Autodesk Inventor part; units mm, degrees
ref_plane "YZ Plane" through (0, 0, 0) normal (1, 0, 0) x (0, 1, 0)
ref_plane "XZ Plane" through (0, 0, 0) normal (0, 1, 0) x (-1, 0, 0)
ref_plane "XY Plane" through (0, 0, 0) normal (0, 0, 1) x (1, 0, 0)
sketch "Sketch1" plane through (0, 0, 0) normal (0, 0, 1) x (1, 0, 0)
  line L0 (17, 4.5) -> (17, -4.5)
  line L1 (-17, -4.5) -> (-17, 4.5)
  arc A0 (-8.3666, -4.5) -> (8.3666, -4.5) centre (0, 0) ccw
  arc A1 (8.3666, 4.5) -> (-8.3666, 4.5) centre (0, 0) ccw
  line L2 (-17, 4.5) -> (-8.3666, 4.5)
  line L3 (8.3666, 4.5) -> (17, 4.5)
  line L4 (17, -4.5) -> (8.3666, -4.5)
  line L5 (-8.3666, -4.5) -> (-17, -4.5)
  line L6 (-17, 4.5) -> (17, -4.5) construction
  line L7 (-17, -4.5) -> (17, 4.5) construction
  point P0 (0, 0)
  point P1 (0, 0)
  dimension "d0" = 9
  dimension "d1" = 34
  dimension "d2" = 9.5
  dimension "d3" = 9
  dimension "d4" = 9.5
  dimension "d12" = 4.5
extrude "Extrusion1" add sketch "Sketch1" along normal blind 7
sketch "Sketch2" plane through (17, -4.5, 0) normal (1, 0, 0) x (0, 0, -1)
  arc A0 (-11.5, 9) -> (-11.5, 0) centre (-11.5, 4.5) ccw
  circle A1 centre (-11.5, 4.5) radius 2.25
  line L0 (-7, 9) -> (-11.5, 9)
  line L1 (-11.5, 0) -> (-7, 0)
  line L2 (-7, 0) -> (-7, 9)
  point P0 (0, 4.5)
  point P1 (-7, 0)
  dimension "d7" = 9
  dimension "d8" = 4.5
  dimension "d9" = 9
extrude "Extrusion2" add sketch "Sketch2" against normal blind 4.3
extrude "Extrusion3" add sketch "Sketch2" along normal blind 4.3 from surface at -34
sketch "Sketch3" plane through (-17, -4.5, 0) normal (0, -1, 0) x (1, 0, 0)
  line L0 (0, 6) -> (0, 0)
  line L1 (0, 0) -> (5, 0)
  line L2 (5, 0) -> (0, 6)
  line L3 (29, 0) -> (34, 0)
  line L4 (34, 0) -> (34, 6)
  line L5 (34, 6) -> (29, 0)
  point P0 (17, 0)
  dimension "d15" = 6
  dimension "d16" = 5
  dimension "d17" = 6
  dimension "d18" = 5
extrude "Extrusion4" cut sketch "Sketch3" against normal up to next
sketch "Sketch4" plane through (0, 0, 0) normal (0, 0, -1) x (-1, 0, 0)
  circle A0 centre (0, 0) radius 7.5
  dimension "d21" = 15
extrude "Extrusion5" add sketch "Sketch4" along normal blind 2.5
sketch "Sketch5" plane through (0, 0, 7) normal (0, 0, 1) x (1, 0, 0)
  circle A0 centre (0, 0) radius 7.5
  dimension "d24" = 15
extrude "Extrusion6" cut sketch "Sketch5" against normal blind 4
sketch "Sketch6" plane through (0, 0, -2.5) normal (0, 0, -1) x (-1, 0, 0)
  circle A0 centre (0, 0) radius 5.5
  dimension "d27" = 11
extrude "Extrusion7" cut sketch "Sketch6" against normal blind 4
sketch "Sketch7" plane through (0, 0, 1.5) normal (0, 0, -1) x (-1, 0, 0)
  circle A0 centre (0, 0) radius 5
  dimension "d30" = 10
extrude "Extrusion8" cut sketch "Sketch7" against normal up to next
sketch "Sketch9" plane through (0, 0, 0) normal (1, 0, 0) x (0, 1, 0)
  arc A0 (31.2893, 14.3034) -> (30.2107, 19.6966) centre (30.75, 17) ccw
  line L0 (-9.5504, 0) -> (57.3026, 0)
  line L1 (0, -37.6235) -> (0, 29.8791)
  circle A1 centre (30.75, 17) radius 1.25
  arc A2 (25.2107, 18.6966) -> (23.9154, 18.0486) centre (25.75, 16) ccw
  circle A3 centre (25.75, 16) radius 1.25
  line L2 (9.5, 7) -> (9.5, 0)
  line L3 (9.5, 0) -> (12.3425, 0)
  line L4 (25.2107, 18.6966) -> (30.2107, 19.6966)
  line L5 (26.2893, 13.3034) -> (31.2893, 14.3034)
  arc A4 (23.9154, 18.0486) -> (9.5, 7) centre (47.7522, -27.9802) ccw
  arc A5 (26.2893, 13.3034) -> (14.061, 0.9769) centre (44.8843, -17.3723) ccw
  arc A6 (12.3425, 0) -> (14.061, 0.9769) centre (12.3425, 2) ccw
  line L6 (8.5, 7) -> (9.5, 7)
  line L7 (9.5, 7) -> (9.5, 0)
  line L8 (9.5, 0) -> (8.5, 0)
  line L9 (8.5, 0) -> (8.5, 7)
  point P0 (0, 0)
  point P1 (13.5, 0)
  dimension "d53" = 5.5
  dimension "d54" = 17
  dimension "d55" = 30.75
  dimension "d56" = 2.5
  dimension "d57" = 16
  dimension "d58" = 25.75
  dimension "d59" = 4
  dimension "d60" = 7
  dimension "d61" = 9.5
  dimension "d62" = 0
  dimension "d63" = 51.8348
  dimension "d64" = 35.8716
  dimension "d65" = 2
  dimension "d88" = 7
  dimension "d89" = 1
  dimension "d90" = 0
  dimension "d91" = 0
extrude "Extrusion9" add sketch "Sketch9" along normal mid plane 4 contours L5 A5 A6 L0 L2 A4 A2 L4 A0
sketch "Sketch10" plane through (0, 0, 0) normal (1, 0, 0) x (0, 1, 0)
  arc A0 (25.2107, 18.6966) -> (26.2893, 13.3034) centre (25.75, 16) ccw
  circle A1 centre (25.75, 16) radius 1.25
  arc A2 (31.2893, 14.3034) -> (30.2107, 19.6966) centre (30.75, 17) ccw
  circle A3 centre (25.75, 16) radius 1.25
  circle A4 centre (30.75, 17) radius 1.25
  circle A5 centre (30.75, 17) radius 1.25
  line L0 (25.2107, 18.6966) -> (30.2107, 19.6966)
  line L1 (26.2893, 13.3034) -> (31.2893, 14.3034)
  point P0 (0, 0)
  dimension "d68" = 5.5
  dimension "d69" = 2.5
extrude "Extrusion10" add sketch "Sketch10" against normal blind 3.5
sketch "Sketch11" plane through (0, 0, 0) normal (1, 0, 0) x (0, 1, 0)
  line L0 (-4.2102, 0) -> (25.2612, 0)
  line L1 (0, -2.5102) -> (0, 15.0612)
  line L2 (19.9196, 12.551) -> (11.6686, 4.3)
  line L3 (11.6686, 4.3) -> (0, 4.3)
  line L4 (21.051, 11.4196) -> (12.3314, 2.7)
  line L5 (12.3314, 2.7) -> (0, 2.7)
  line L6 (21.051, 11.4196) -> (19.9196, 12.551)
  line L7 (0, 4.3) -> (0, 2.7)
  point P0 (0, 0)
extrude "Extrusion11" add sketch "Sketch11" along normal mid plane 12
extrude "Extrusion12" cut sketch "Sketch5" against normal blind 4
extrude "Extrusion13" cut sketch "Sketch7" against normal through all
sketch "Sketch12" plane through (0, 0, 0) normal (0, 0, 1) x (1, 0, 0)
  line L0 (6, 7.3655) -> (6, 12.3314)
  line L1 (2, 21.051) -> (6, 21.051)
  arc A0 (6, 7.3655) -> (2, 21.051) centre (-49.0316, -1.2919) ccw
  line L2 (0, 0) -> (0, 16.5543) construction
  arc A1 (-2, 21.051) -> (-6, 7.3655) centre (49.0316, -1.2919) ccw
  line L3 (2, 26.2893) -> (2, 14.061) construction
  line L4 (2, 21.051) -> (6, 21.051)
  line L5 (6, 7.3655) -> (6, 21.051)
  line L6 (-6, 7.3655) -> (-6, 21.051)
  line L7 (-2, 21.051) -> (-6, 21.051)
extrude "Extrusion14" cut sketch "Sketch12" along normal up to next
sketch "Sketch13" plane through (0, 0, 0) normal (1, 0, 0) x (0, 1, 0)
  line L0 (8.5, 7) -> (9.5, 7)
  line L1 (9.5, 7) -> (9.5, 0)
  line L2 (9.5, 0) -> (8.5, 0)
  line L3 (8.5, 0) -> (8.5, 7)
  line L4 (0, -6.95) -> (0, 24.2)
  line L5 (-18.1, 0) -> (42.1, 0)
  point P0 (0, 0)
  dimension "d92" = 7
  dimension "d93" = 1
  dimension "d94" = 9.5
  dimension "d95" = 0
extrude "Extrusion15" add sketch "Sketch13" along normal mid plane 4
properties part number "RCT-P006_steering_knuckle"
Geometry check sheet. Reference: the model listing, model coordinates, mm. A direction names the side the tool comes from. Coordinates: 2 decimals unless noted, no trailing zeros. Loops run counter-clockwise (first coordinate to the right, second up) from the corner with the lowest first, then second, coordinate; pieces in that order, holes last. Notation, with made-up numbers: (57.25, 17) - (107.25, 17) arc R24 ccw to (107.25, 49) - close; hole circle Ø9 at (-16.75, -16). An arc over 180 degrees is marked (long way). One line per item, written item: value. Start each with the question number.
(1) Tool access check on faces 1 (the cylindrical face through (-6.454, 6.971, 3.451)), 2 (the flat face through (-13, 4.5, 6)), 3 (the flat face through (6, 5, 0)), 4 (the flat face through (13, 4.5, 6)), 5 (the flat face through (-3.25, 14.94, 7.57)). Record the directions out of +Z, -Z, +X, -X, +Y, -Y that give a thin tool (end or side, any length) a straight path to the whole face; none if there is none.
(2) Cross-section at C-C on x = -14. Enter the section's corners in (y, z), plus the area to 3 significant figures.
(3) Material ranges on line 1 (Y direction, x = 0, z = -1); line 2 (Y direction, x = -13.6, z = 11.5); line 3 (X direction, y = 1.5, z = 8.5), recorded low to high. Write a range as [from, to].
(4) Cross-section at D-D on y = 25.75. Enter the section's corners in (x, z).
(5) Cross-section at B-B on x = 0. Enter the section's corners in (y, z).
(6) Mould release check, pull along Y, two halves, no side actions. Record for faces 6 (the cylindrical face through (-0.788, 26.422, 14.946)), 7 (the cylindrical face through (4.279, 14.876, 6.873)), 8 (the flat face through (-0.71, 27.68, 19.19)): released by +Y, released by -Y, zero draft, split by the parting line, or undercut.
(7) Cross-section at A-A on y = 0. Count the separate pieces of the cut face and the enclosed holes in it, plus the area to 3 significant figures.
(8) Depth check by flat-ended pin: P1, Ø10, axis at x = 2.5, z = 16.5, coming from the -Y side; P2, Ø12, axis at y = 25, z = 16, coming from the +X side; P3, Ø7, axis at x = -12.5, z = 3.5, coming from the +Y side. Enter the tip coordinate at first touch or a pass-through.
Results below:
1. face 1: -X
1. face 2: +Z, -Z, -X, +Y
1. face 3: -Z
1. face 4: +Z, -Z, +X, +Y
1. face 5: +Z, -X
2. outline: (-4.5, 2.4) - (4.5, 2.4) - (4.5, 11.5) arc R4.5 ccw to (-4.5, 11.5) - close; hole circle Ø4.5 at (0, 11.5)
2. area: 97.8 mm2
3. line 1: y = [-7.5, -5.5], [5.5, 7.5]
3. line 2: y = [-4.5, -2.25], [2.25, 4.5]
3. line 3: x = [-17, -12.7], [12.7, 17]
4. outline: (-3.5, 13.25) - (-2, 13.25) - (-2, 12.97) - (2, 12.97) - (2, 14.75) - (-3.5, 14.75) - close; (-3.5, 17.25) - (2, 17.25) - (2, 18.8) - (-3.5, 18.8) - close
5. outline: (-9.5, 0) - (-7.5, 0) - (-7.5, -2.5) - (-5.5, -2.5) - (-5.5, 1.5) - (-5, 1.5) - (-5, 3) - (-7.5, 3) - (-7.5, 7) - (-9.5, 7) - close; (5, 1.5) - (5.5, 1.5) - (5.5, -2.5) - (7.5, -2.5) - (7.5, 0) - (12.34, 0) arc R2 ccw to (14.06, 0.98) arc R35.87 cw to (26.29, 13.3) - (31.29, 14.3) arc R2.75 ccw to (30.21, 19.7) - (25.21, 18.7) arc R2.75 ccw to (23.92, 18.05) arc R51.84 ccw to (9.5, 7) - (7.5, 7) - (7.5, 3) - (5, 3) - close; hole circle Ø2.5 at (25.75, 16); hole circle Ø2.5 at (30.75, 17)
6. face 6: undercut
6. face 7: released by +Y
6. face 8: released by -Y
7. separate pieces: 4
7. enclosed holes: 0
7. area: 165 mm2
8. P1: stops at y = 14.19
8. P2: stops at x = 2
8. P3: stops at y = 4.5
